Check sheet for the modelled part. Datum: model origin and axes. Units: mm. Coordinates: 2 decimals unless noted, no trailing zeros. Write each loop counter-clockwise with the first axis right and the second up, starting at its lowest first coordinate (ties: lowest second). Pieces come first, ordered by that corner, then holes. Notation, with made-up numbers: (-27.5, -12) - (21.5, -12) arc R16 ccw to (21.5, -8) - close; hole circle Ø9 at (52.5, -6.75). An arc over 180 degrees is marked (long way). Write each question's results on one line, items separated by ' | '.
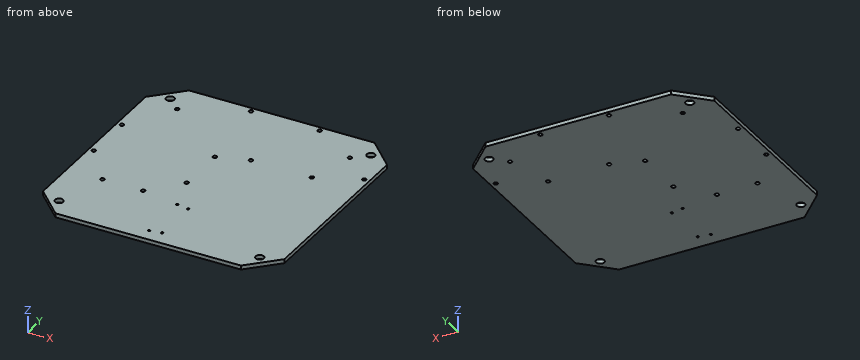
Autodesk Inventor part; units mm, degrees
ref_plane "Zplus_face" through (0, 0, 1.5875) normal (0, 0, 1) x (1, 0, 0)
ref_plane "Work Plane_ConnX" through (-32, 0, 0) normal (1, 0, 0) x (0, 1, 0)
ref_plane "Work Plane_ConnY" through (0, 0, 0) normal (0, 1, 0) x (-1, 0, 0)
sketch "AL_spacer_contact_Zminus" plane through (0, 0, 0) normal (0, 0, 1) x (1, 0, 0)
  circle A0 centre (39.5, 39.5) radius 3.175
  circle A1 centre (39.5, -39.5) radius 3.175
  circle A2 centre (-39.5, -39.5) radius 3.175
  circle A3 centre (-39.5, 39.5) radius 3.175
  point P0 (0, 0)
  dimension "d228" = 39.5
  dimension "d229" = 39.5
  dimension "d230" = 39.5
  dimension "d231" = 39.5
  dimension "d232" = 39.5
  dimension "d233" = 39.5
  dimension "d234" = 39.5
  dimension "d235" = 39.5
  dimension "d236" = 6.35
sketch "Delrin_stayout_Zminus" plane through (0, 0, 0) normal (0, 0, 1) x (1, 0, 0)
  line L0 (47.5, 39.5) -> (47.5, 31)
  line L1 (47.5, 31) -> (39.5, 31)
  line L2 (39.5, 31) -> (31, 39.5)
  line L3 (31, 39.5) -> (31, 47.5)
  line L4 (31, 47.5) -> (39.5, 47.5)
  line L5 (39.5, 47.5) -> (47.5, 39.5)
  line L6 (-39.5, 47.5) -> (-47.5, 39.5)
  line L7 (-47.5, 39.5) -> (-47.5, 31)
  line L8 (-47.5, 31) -> (-39.5, 31)
  line L9 (-39.5, 31) -> (-31, 39.5)
  line L10 (-31, 39.5) -> (-31, 47.5)
  line L11 (-31, 47.5) -> (-39.5, 47.5)
  line L12 (47.5, -39.5) -> (39.5, -47.5)
  line L13 (39.5, -47.5) -> (31, -47.5)
  line L14 (31, -47.5) -> (31, -39.5)
  line L15 (31, -39.5) -> (39.5, -31)
  line L16 (39.5, -31) -> (47.5, -31)
  line L17 (47.5, -31) -> (47.5, -39.5)
  line L18 (-39.5, -47.5) -> (-47.5, -39.5)
  line L19 (-47.5, -39.5) -> (-47.5, -31)
  line L20 (-47.5, -31) -> (-39.5, -31)
  line L21 (-39.5, -31) -> (-31, -39.5)
  line L22 (-31, -39.5) -> (-31, -47.5)
  line L23 (-31, -47.5) -> (-39.5, -47.5)
  point P0 (0, 0)
  dimension "d243" = 16.5
  dimension "d244" = 8
  dimension "d245" = 8.5
  dimension "d246" = 16.5
  dimension "d247" = 47.5
  dimension "d248" = 47.5
  dimension "d249" = 47.5
  dimension "d250" = 47.5
  dimension "d251" = 47.5
  dimension "d252" = 47.5
  dimension "d253" = 47.5
  dimension "d254" = 47.5
sketch "Nub_stayout_Zminus" plane through (0, 0, 0) normal (0, 0, 1) x (1, 0, 0)
  line L0 (29, 47.5) -> (39.5, 47.5)
  line L1 (39.5, 47.5) -> (47.5, 39.5)
  line L2 (47.5, 39.5) -> (47.5, 29)
  line L3 (47.5, 29) -> (42, 29)
  line L4 (42, 29) -> (42, 40.4125)
  line L5 (40.4125, 42) -> (29, 42)
  line L6 (29, 42) -> (29, 47.5)
  arc A0 (42, 40.4125) -> (40.4125, 42) centre (40.4125, 40.4125) ccw
  line L7 (-29, 47.5) -> (-39.5, 47.5)
  line L8 (-39.5, 47.5) -> (-47.5, 39.5)
  line L9 (-47.5, 39.5) -> (-47.5, 29)
  line L10 (-47.5, 29) -> (-42, 29)
  line L11 (-42, 29) -> (-42, 40.4125)
  line L12 (-40.4125, 42) -> (-29, 42)
  line L13 (-29, 42) -> (-29, 47.5)
  arc A1 (-40.4125, 42) -> (-42, 40.4125) centre (-40.4125, 40.4125) ccw
  line L14 (-47.5, -29) -> (-42, -29)
  line L15 (-42, -29) -> (-42, -40.4125)
  line L16 (-40.4125, -42) -> (-29, -42)
  line L17 (-29, -42) -> (-29, -47.5)
  line L18 (-29, -47.5) -> (-39.5, -47.5)
  line L19 (-39.5, -47.5) -> (-47.5, -39.5)
  line L20 (-47.5, -39.5) -> (-47.5, -29)
  arc A2 (-42, -40.4125) -> (-40.4125, -42) centre (-40.4125, -40.4125) ccw
  line L21 (47.5, -29) -> (42, -29)
  line L22 (42, -29) -> (42, -40.4125)
  line L23 (40.4125, -42) -> (29, -42)
  line L24 (29, -42) -> (29, -47.5)
  line L25 (29, -47.5) -> (39.5, -47.5)
  line L26 (39.5, -47.5) -> (47.5, -39.5)
  line L27 (47.5, -39.5) -> (47.5, -29)
  arc A3 (40.4125, -42) -> (42, -40.4125) centre (40.4125, -40.4125) ccw
  point P0 (0, 0)
  dimension "d255" = 1.5875
  dimension "d256" = 18.5
  dimension "d257" = 8
  dimension "d258" = 5.5
  dimension "d259" = 47.5
  dimension "d260" = 47.5
  dimension "d264" = 1.5875
  dimension "d265" = 47.5
  dimension "d266" = 47.5
  dimension "d267" = 1.5875
  dimension "d268" = 47.5
  dimension "d269" = 47.5
  dimension "d270" = 1.5875
  dimension "d271" = 47.5
  dimension "d272" = 47.5
ref_plane "Zplus_face" through (0, 0, 1.5875) normal (0, 0, 1) x (1, 0, 0)
sketch "AL_spacer_contact_Zplus" plane through (0, 0, 1.5875) normal (0, 0, 1) x (1, 0, 0)
  circle A0 centre (-39.5, 39.5) radius 3.175
  circle A1 centre (-39.5, -39.5) radius 3.175
  circle A2 centre (39.5, -39.5) radius 3.175
  circle A3 centre (39.5, 39.5) radius 3.175
  point P0 (0, 0)
  dimension "d129" = 39.5
  dimension "d130" = 39.5
  dimension "d131" = 39.5
  dimension "d132" = 39.5
  dimension "d133" = 6.35
sketch "Delrin_stayout_Zplus" plane through (0, 0, 1.5875) normal (0, 0, 1) x (1, 0, 0)
  line L0 (47.5, -31) -> (47.5, -39.5)
  line L1 (47.5, -39.5) -> (39.5, -47.5)
  line L2 (39.5, -47.5) -> (31, -47.5)
  line L3 (31, -47.5) -> (31, -39.5)
  line L4 (31, -39.5) -> (39.5, -31)
  line L5 (39.5, -31) -> (47.5, -31)
  line L6 (47.5, 31) -> (47.5, 39.5)
  line L7 (47.5, 39.5) -> (39.5, 47.5)
  line L8 (39.5, 47.5) -> (31, 47.5)
  line L9 (31, 47.5) -> (31, 39.5)
  line L10 (31, 39.5) -> (39.5, 31)
  line L11 (39.5, 31) -> (47.5, 31)
  line L12 (-39.5, 47.5) -> (-47.5, 39.5)
  line L13 (-47.5, 39.5) -> (-47.5, 31)
  line L14 (-47.5, 31) -> (-39.5, 31)
  line L15 (-39.5, 31) -> (-31, 39.5)
  line L16 (-31, 39.5) -> (-31, 47.5)
  line L17 (-31, 47.5) -> (-39.5, 47.5)
  line L18 (-47.5, -39.5) -> (-39.5, -47.5)
  line L19 (-39.5, -47.5) -> (-31, -47.5)
  line L20 (-31, -47.5) -> (-31, -39.5)
  line L21 (-31, -39.5) -> (-39.5, -31)
  line L22 (-39.5, -31) -> (-47.5, -31)
  line L23 (-47.5, -31) -> (-47.5, -39.5)
  point P0 (0, 0)
  dimension "d115" = 16.5
  dimension "d116" = 16.5
  dimension "d117" = 8
  dimension "d118" = 8.5
  dimension "d121" = 47.5
  dimension "d122" = 47.5
  dimension "d123" = 47.5
  dimension "d124" = 47.5
  dimension "d125" = 47.5
  dimension "d126" = 47.5
  dimension "d127" = 47.5
  dimension "d128" = 47.5
sketch "Nub_stayout_Zplus" plane through (0, 0, 1.5875) normal (0, 0, 1) x (1, 0, 0)
  line L0 (47.5, 29) -> (42, 29)
  line L1 (42, 29) -> (42, 40.4125)
  line L2 (40.4125, 42) -> (29, 42)
  line L3 (29, 42) -> (29, 47.5)
  arc A0 (42, 40.4125) -> (40.4125, 42) centre (40.4125, 40.4125) ccw
  line L4 (29, 47.5) -> (39.5, 47.5)
  line L5 (39.5, 47.5) -> (47.5, 39.5)
  line L6 (47.5, 39.5) -> (47.5, 29)
  line L7 (-39.5, 47.5) -> (-29, 47.5)
  line L8 (-29, 47.5) -> (-29, 42)
  line L9 (-29, 42) -> (-40.4125, 42)
  line L10 (-42, 40.4125) -> (-42, 29)
  line L11 (-42, 29) -> (-47.5, 29)
  line L12 (-47.5, 29) -> (-47.5, 39.5)
  line L13 (-47.5, 39.5) -> (-39.5, 47.5)
  arc A1 (-40.4125, 42) -> (-42, 40.4125) centre (-40.4125, 40.4125) ccw
  line L14 (-47.5, -29) -> (-47.5, -39.5)
  line L15 (-47.5, -39.5) -> (-39.5, -47.5)
  line L16 (-39.5, -47.5) -> (-29, -47.5)
  line L17 (-29, -47.5) -> (-29, -42)
  line L18 (-29, -42) -> (-40.4125, -42)
  line L19 (-42, -40.4125) -> (-42, -29)
  line L20 (-42, -29) -> (-47.5, -29)
  arc A2 (-42, -40.4125) -> (-40.4125, -42) centre (-40.4125, -40.4125) ccw
  line L21 (29, -47.5) -> (39.5, -47.5)
  line L22 (39.5, -47.5) -> (47.5, -39.5)
  line L23 (47.5, -39.5) -> (47.5, -29)
  line L24 (47.5, -29) -> (42, -29)
  line L25 (42, -29) -> (42, -40.4125)
  line L26 (40.4125, -42) -> (29, -42)
  line L27 (29, -42) -> (29, -47.5)
  arc A3 (40.4125, -42) -> (42, -40.4125) centre (40.4125, -40.4125) ccw
  point P0 (0, 0)
  dimension "d146" = 1.5875
  dimension "d147" = 5.5
  dimension "d149" = 18.5
  dimension "d150" = 8
  dimension "d151" = 47.5
  dimension "d152" = 47.5
  dimension "d153" = 1.5875
  dimension "d154" = 47.5
  dimension "d155" = 47.5
  dimension "d156" = 1.5875
  dimension "d157" = 47.5
  dimension "d158" = 47.5
  dimension "d159" = 1.5875
  dimension "d160" = 47.5
  dimension "d161" = 47.5
sketch "Sketch1" plane through (0, 0, 0) normal (0, 0, 1) x (1, 0, 0)
  line L0 (-47.5, 47.5) -> (47.5, 47.5)
  line L1 (47.5, 47.5) -> (47.5, -47.5)
  line L2 (47.5, -47.5) -> (-47.5, -47.5)
  line L3 (-47.5, -47.5) -> (-47.5, 47.5)
  point P0 (0, 0)
  dimension "d0" = 95
  dimension "d1" = 95
  dimension "d2" = 47.5
  dimension "d3" = 47.5
extrude "Extrusion1" add sketch "Sketch1" along normal blind 1.5875
chamfer "Chamfer2" distance 11 angle 45 4 edges at (-47.5, -47.5, 0.7937) (47.5, -47.5, 0.7937) (47.5, 47.5, 0.7937) (-47.5, 47.5, 0.7937)
ref_plane "Work Plane_ConnX" through (-32, 0, 0) normal (1, 0, 0) x (0, 1, 0)
ref_plane "Work Plane_ConnY" through (0, 0, 0) normal (0, 1, 0) x (-1, 0, 0)
sketch "Sketch9" plane through (0, 0, 1.5875) normal (0, 0, 1) x (1, 0, 0)
  line L0 (47.5, 47.5) -> (47.5, -47.5)
  line L1 (58.5598, -32) -> (-58.5598, -32)
  circle A0 centre (-2.667, -21.9289) radius 0.4445
  circle A1 centre (-2.667, -42.0711) radius 0.4445
  line L2 (0, 26.5598) -> (0, -90.5598) construction
  point P0 (0, 0)
  point P1 (0, -32)
  dimension "d134" = 20.1422
  dimension "d136" = 2.667
  dimension "d138" = 0.889
  dimension "d141" = 180
  dimension "d350" = 32
  dimension "d351" = 0
extrude "Holes_Conn_Zminus" cut sketch "Sketch9" against normal through all
sketch "Sketch22" plane through (0, 0, 1.5875) normal (0, 0, 1) x (1, 0, 0)
  line L0 (47.5, 36.5) -> (47.5, -36.5)
  line L1 (0, -1.0026) -> (0, -62.9974) construction
  line L2 (62.8115, -32) -> (-62.8115, -32)
  circle A0 centre (2.032, -22.7545) radius 0.4445
  circle A1 centre (2.032, -41.2455) radius 0.4445
  point P0 (0, 0)
  point P1 (0, -32)
  dimension "d282" = 180
  dimension "d283" = 18.491
  dimension "d284" = 0.889
  dimension "d285" = 2.032
  dimension "d352" = 32
  dimension "d353" = 0
extrude "Holes_Conn_Zplus" cut sketch "Sketch22" against normal through all
hole "Hole5" at (39.5, 39.5, 1.5875) direction (0, 0, -1) diameter 3.2 end through all
mirror "Mirror5" about plane through (0, 0, 0) normal (1, 0, 0) of "Hole5"
mirror "Mirror6" about plane through (0, 0, 0) normal (0, 1, 0) of "Hole5", "Mirror5"
sketch "Sketch25" plane through (0, 0, 1.5875) normal (0, 0, 1) x (1, 0, 0)
  circle A0 centre (-39.5, -39.5) radius 1.6
  circle A1 centre (39.5, -39.5) radius 1.6
  circle A2 centre (-39.5, 39.5) radius 1.6
  circle A3 centre (39.5, 39.5) radius 1.6
  line L0 (36.5, -47.5) -> (-36.5, -47.5)
  line L1 (0, 0) -> (0, -59.2198)
  line L2 (8, -47.5) -> (8, -15.5)
  line L3 (8, -15.5) -> (-8, -15.5)
  line L4 (-8, -15.5) -> (-8, -47.5)
  line L5 (-8, -47.5) -> (-62.7516, -61.7336)
  line L6 (-62.7516, -61.7336) -> (-64.2933, 68.2222)
  line L7 (-64.2933, 68.2222) -> (58.3572, 62.5728)
  line L8 (58.3572, 62.5728) -> (56.5848, -69.017)
  line L9 (56.5848, -69.017) -> (8, -47.5)
  dimension "d362" = 16
  dimension "d363" = 32
extrude "Extrusion9" [suppressed]
sketch "Sketch27" plane through (0, 0, 0) normal (0, 0, -1) x (-1, 0, 0)
  line L0 (36.5, 47.5) -> (-36.5, 47.5)
  line L1 (-47.5, 36.5) -> (-47.5, -36.5)
  line L2 (-36.5, -47.5) -> (36.5, -47.5)
  line L3 (47.5, -36.5) -> (47.5, 36.5)
  line L4 (-47.5, 47.5) -> (47.5, 47.5) construction
  line L5 (47.5, 47.5) -> (47.5, -47.5) construction
  line L6 (47.5, -47.5) -> (-47.5, -47.5) construction
  line L7 (-47.5, -47.5) -> (-47.5, 47.5) construction
  point P0 (0, 0)
decal "Decal2"
sketch "Sketch29" plane through (0, 0, 1.5875) normal (0, 0, 1) x (1, 0, 0)
  line L0 (-47.5, -36.5) -> (-47.5, 36.5)
  line L1 (36.5, -47.5) -> (-36.5, -47.5)
  line L2 (47.5, 36.5) -> (47.5, -36.5)
  line L3 (-36.5, 47.5) -> (36.5, 47.5)
  line L4 (-47.5, 47.5) -> (47.5, 47.5) construction
  line L5 (47.5, 47.5) -> (47.5, -47.5) construction
  line L6 (47.5, -47.5) -> (-47.5, -47.5) construction
  line L7 (-47.5, -47.5) -> (-47.5, 47.5) construction
  point P0 (0, 0)
decal "Decal3"
ref_plane "U7_MBC13917_X" through (4.5, -36.5, 0) normal (-1, 0, 0) x (0, 0, 1)
ref_plane "U7_MBC13917_Y" through (-36.5, 42.03, 0) normal (0, -1, 0) x (1, 0, 0)
ref_plane "U9_SA601_X" through (-23.16, -36.5, 0) normal (-1, 0, 0) x (0, 0, 1)
ref_plane "U9_SA601_Y" through (-36.5, 37.32, 0) normal (0, -1, 0) x (1, 0, 0)
ref_plane "U10_SA607_X" through (-18, -36.5, 0) normal (-1, 0, 0) x (0, 0, 1)
ref_plane "U10_SA607_Y" through (-36.5, 4, 0) normal (0, -1, 0) x (1, 0, 0)
hole "Hole13" at (-17.5, -19.5, 1.5875) direction (0, 0, -1) diameter 1.6 end through all
hole "Hole14" at (-7, -7.5, 1.5875) direction (0, 0, -1) diameter 1.6 end through all
hole "Hole15" at (-7, 12.5, 1.5875) direction (0, 0, -1) diameter 1.6 end through all
hole "Hole16" at (5, 16.5, 1.5875) direction (0, 0, -1) diameter 1.6 end through all
hole "Hole17" at (16, 45.5, 1.5875) direction (0, 0, -1) diameter 1.6 end through all
hole "Hole18" at (34, 34.5, 1.5875) direction (0, 0, -1) diameter 1.6 end through all
hole "Hole19" at (45.5, 24, 1.5875) direction (0, 0, -1) diameter 1.6 end through all
hole "Hole20" at (29, 16.5, 1.5875) direction (0, 0, -1) diameter 1.6 end through all
hole "Hole21" at (-11, 45.5, 1.5875) direction (0, 0, -1) diameter 1.6 end through all
hole "Hole22" at (-34, 34.5, 1.5875) direction (0, 0, -1) diameter 1.6 end through all
hole "Hole23" at (-45.5, 16, 1.5875) direction (0, 0, -1) diameter 1.6 end through all
hole "Hole24" at (-45.5, -4, 1.5875) direction (0, 0, -1) diameter 1.6 end through all
hole "Hole25" at (-33.5, -19.5, 1.5875) direction (0, 0, -1) diameter 1.6 end through all
properties part number "PCB_RX" material "FR4"
1. Sectioned sample at B-B (z = 0.35). Give the number of separate pieces and of enclosed holes in the cut face, then the cut area to 3 significant figures.
Values follow:
separate pieces: 1 | enclosed holes: 21 | area: 8,720 mm^2
2. Material ranges on L1, parallel to X at y = -19.5, z = 0.55; L2, parallel to X at y = 34.5, z = 1.3; L3, parallel to X at y = -4, z = 1.35, recorded low to high. Write a range as [from, to].
Values follow:
L1: x = [-47.5, -34.3], [-32.7, -18.3], [-16.7, 47.5] | L2: x = [-47.5, -34.8], [-33.2, 33.2], [34.8, 47.5] | L3: x = [-47.5, -46.3], [-44.7, 47.5]
3. Sectioned sample at A-A (x = -39.5). Record the cut outline in (y, z), then the cut area to 3 significant figures.
Values follow:
outline: (-44.5, 0) - (-41.1, 0) - (-41.1, 1.59) - (-44.5, 1.59) - close; (-37.9, 0) - (37.9, 0) - (37.9, 1.59) - (-37.9, 1.59) - close; (41.1, 0) - (44.5, 0) - (44.5, 1.59) - (41.1, 1.59) - close | area: 131 mm^2
